```python
from build123d import *

# Parameters (mm, degrees)
SKETCH011_R          = 27.5
SKETCH011_R_2        = 25.5
PAD001_DEPTH         = 25
CHAMFER002_SIZE2     = 1
CHAMFER002_SIZE      = 10
CHAMFER002_FACE3_R   = 27.5
CHAMFER002_FACE3_R_2 = 25.5
PAD002_DEPTH         = 3
SKETCH012_R          = 29
SKETCH012_R_2        = 25.5
PAD003_DEPTH         = 1


with BuildPart() as part:
    # Sketch011 (on Face1 of CopyChamfer001) → Pad001 (new body)
    with BuildSketch(Plane.XY.offset(72)):
        with Locations((0, 80)):
            Circle(SKETCH011_R)
        with Locations((0, 80)):
            Circle(SKETCH011_R_2, mode=Mode.SUBTRACT)
    extrude(amount=PAD001_DEPTH)

    # Chamfer002
    chamfer002_edges = [part.edges().sort_by_distance(p)[0] for p in [
        (-27.5, 80, 97),
    ]]
    chamfer002_side = part.faces().sort_by_distance((-27.5, 80, 84.5))[0]
    chamfer(chamfer002_edges, length=CHAMFER002_SIZE, length2=CHAMFER002_SIZE2, reference=chamfer002_side)

    # Chamfer002 Face3 → Pad002 (add)
    with BuildSketch(Plane(origin=(0, 80, 72), x_dir=(0, -1, 0), z_dir=(0, 0, -1))):
        Circle(CHAMFER002_FACE3_R)
        Circle(CHAMFER002_FACE3_R_2, mode=Mode.SUBTRACT)
    extrude(amount=PAD002_DEPTH)

    # Sketch012 (on Face5 of Pad002) → Pad003 (join)
    with BuildSketch(Plane(origin=(0, 0, 69), x_dir=(1, 0, 0), z_dir=(0, 0, -1))):
        with Locations((0, -80)):
            Circle(SKETCH012_R)
        with Locations((0, -80)):
            Circle(SKETCH012_R_2, mode=Mode.SUBTRACT)
    extrude(amount=PAD003_DEPTH)


solid = part.part
```
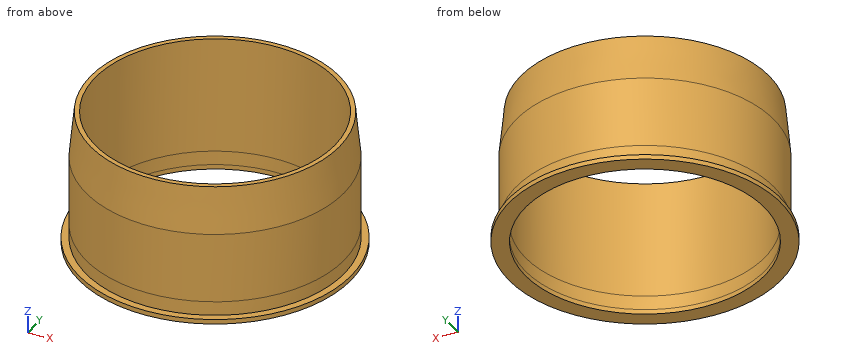
CAD build for the part. Positions are in the model's coordinates, mm. Coordinates: 2 decimals unless noted, no trailing zeros. Write each loop counter-clockwise with the first axis right and the second up, starting at its lowest first coordinate (ties: lowest second). Pieces come first, ordered by that corner, then holes. Notation, with made-up numbers: (35, 74.5) -> (68, 74.5) arc R13 ccw to (68, 86.5) -> close; hole circle Ø2 at (58, -30.5). An arc over 180 degrees is marked (long way). Use CSV: the item, a comma, the result in double quotes. Start each with the question number.
Item 1: Band-saw the part on B-B, the plane y = 80. Write the cut outline in (x, z).
Item 2: Wall check: probe 1 along Y at (x, z) = (0, 71); probe 2 along X at (y, z) = (80, 68.45); probe 3 along X at (y, z) = (80, 70.4). Give the ranges that are in metal, low to high.
Item 3: Drop flat-ended pins along their axis: P1, Ø5, axis at y = 65, z = 83, coming from the -X side; P2, Ø5, axis at x = 18.5, y = 68, coming from the -Z side; P3, Ø12, axis at y = 90.5, z = 72, coming from the -X side; P4, Ø1.5, axis at x = -21.5, z = 78, coming from the -Y side. Give the stop position or say it passes through.
Item 4: Band-saw the part on C-C, the plane z = 76.5. Write the cut outline in (x, y).
Item 5: Band-saw the part on A-A, the plane x = 0. Write the cut outline in (y, z).
Item 6: Band-saw the part on D-D, the plane z = 88.5. Write the cut outline in (x, y).
Response values:
1,outline,"(-29, 68) -> (-25.5, 68) -> (-25.5, 97) -> (-26.5, 97) -> (-27.5, 87) -> (-27.5, 69) -> (-29, 69) -> close; (25.5, 68) -> (29, 68) -> (29, 69) -> (27.5, 69) -> (27.5, 87) -> (26.5, 97) -> (25.5, 97) -> close"
2,probe 1,"y = 52.5 to 54.5, 105.5 to 107.5"
2,probe 2,"x = -29 to -25.5, 25.5 to 29"
2,probe 3,"x = -27.5 to -25.5, 25.5 to 27.5"
3,P1,"stops at x = -24.49"
3,P2,"passes through"
3,P3,"stops at x = -28.51"
3,P4,"stops at y = 61.95"
4,outline,"circle Ø55 at (0, 80); hole circle Ø51 at (0, 80)"
5,outline,"(51, 68) -> (54.5, 68) -> (54.5, 97) -> (53.5, 97) -> (52.5, 87) -> (52.5, 69) -> (51, 69) -> close; (105.5, 68) -> (109, 68) -> (109, 69) -> (107.5, 69) -> (107.5, 87) -> (106.5, 97) -> (105.5, 97) -> close"
6,outline,"circle Ø54.7 at (0, 80); hole circle Ø51 at (0, 80)"
